Input: part model. Units: mm. Frame: model coordinates. Face numbers are marked on the shaded views. A direction names the side the tool comes from. Round coordinates to 2 decimals unless told otherwise and drop trailing zeros. Loops run counter-clockwise (first coordinate to the right, second up) from the corner with the lowest first, then second, coordinate; pieces in that order, holes last. Notation, with made-up numbers: M -35.5,12.25 L 15.5,12.25 A18 ccw 15.5,24.25 Z; hole C 66,-17.5 d7. An arc over 180 degrees is marked long. Put each result on its own line as item: value. Start each with the question number.
1) Draft query along X for the marked faces 4, 5 and 6. Return one class per face: +X half, -X half, draft (parallel to the pull), parting line (faces both ways), or undercut.
2) Reachability of the marked faces 1, 2 and 3 from +Z, -Z, +X, -X, +Y, -Y: full face, straight path, thin tool, end or side. Return the list, or none.
3) Section B-B on y = -3. Output: boundary loops of the cut face in (x, z).
4) Line query: probe 1 along Z at (x, y) = (25, 2); probe 2 along X at (y, z) = (1.5, -1.25); probe 3 along Y at (x, z) = (0, -3). Output: solid intervals per line, ascending.
5) Pin query (flat end, axial travel): pin 1 (3 mm diameter, centred on x = 12, z = 1.5, fed in from -Y); pin 2 (9.5 mm diameter, centred on x = 52, y = -11, fed in from -Z); pin 3 (2 mm diameter, centred on y = -16, z = 1, fed in from -X); pin 4 (1 mm diameter, centred on x = 76, y = -10, fed in from -Z). Return the tip coordinate at first contact, or that it passes through.
6) Section C-C on x = -25. Output: boundary loops of the cut face in (y, z), plus the area to 3 significant figures.
7) Section A-A on z = 2.5. Output: boundary loops of the cut face in (x, y), plus the area to 3 significant figures.
8) Section D-D on x = 88.5. Output: boundary loops of the cut face in (y, z), plus the area to 3 significant figures.
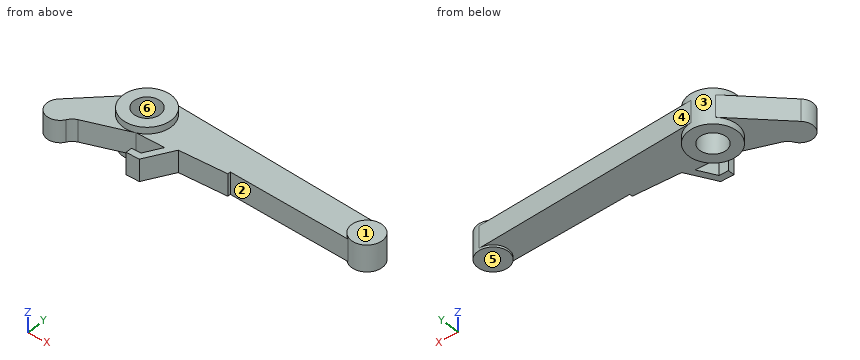
from build123d import *

# Parameters (mm, degrees)
SKETCH1_R               = 11
SKETCH1_R_2             = 6
BOSS_EXTRUDE1_DEPTH     = 8
SKETCH2_R               = 7
BOSS_EXTRUDE2_DEPTH     = 6
BOSS_EXTRUDE3_DEPTH     = 5
CUT_EXTRUDE1_DEPTH      = 112.742355901
CUT_EXTRUDE1_DEPTH_BACK = 112.742355901
SKETCH3_R               = 6


with BuildPart() as part:
    # Sketch1 → Boss-Extrude1 (new, symmetric)
    with BuildSketch(Plane.XY):
        Circle(SKETCH1_R)
        Circle(SKETCH1_R_2, mode=Mode.SUBTRACT)
    extrude(amount=BOSS_EXTRUDE1_DEPTH, both=True)



with BuildPart() as body_2:
    # Sketch2 → Boss-Extrude2 (new, symmetric)
    with BuildSketch(Plane.XY):
        with Locations((102, -3)):
            Circle(SKETCH2_R)
    extrude(amount=BOSS_EXTRUDE2_DEPTH, both=True)


with BuildPart() as part_1:
    add(part.part)

    add(body_2.part)  # Boss-Extrude3 merges body 2
    # Sketch2_3 → Boss-Extrude3 (add, symmetric)
    with BuildSketch(Plane.XY):
        with BuildLine():
            ThreePointArc((0.754140733, 10.974118268), (-3.77780396, 10.330933997), (-7.655588843, 7.898858112))
            Line((-7.655588843, 7.898858112), (-29.175775732, -12.958549415))
            ThreePointArc((-29.175775732, -12.958549415), (-28.687665444, -22), (-19.801298619, -20.262598212))
            ThreePointArc((-19.801298619, -20.262598212), (-18.446505094, -18.651187263), (-16.618471977, -17.606962351))
            Line((-16.618471977, -17.606962351), (3.695770356, -10.360563762))
            Line((3.695770356, -10.360563762), (16.576592604, -10.360563762))
            Line((16.576592604, -10.360563762), (12.165962036, -18))
            Line((12.165962036, -18), (7.898012843, -18))
            Line((7.898012843, -18), (7.898012843, -21))
            Line((7.898012843, -21), (13.898012843, -21))
            Line((13.898012843, -21), (21.138158023, -8.459700694))
            Line((21.138158023, -8.459700694), (42.898012843, -7.651891962))
            Line((42.898012843, -7.651891962), (42.898012843, -6.302949113))
            Line((42.898012843, -6.302949113), (98.5, -9.062177826))
            ThreePointArc((98.5, -9.062177826), (95.304638828, -0.957418601), (102.479907739, 3.983529807))
            Line((102.479907739, 3.983529807), (0.754140733, 10.974118268))
        make_face()
    extrude(amount=BOSS_EXTRUDE3_DEPTH, both=True)

    # Sketch3 → Cut-Extrude1 (cut, two sides: drawn at the far end of the back side and taken through both)
    with BuildSketch(Plane.XY.offset(-CUT_EXTRUDE1_DEPTH_BACK)):
        Circle(SKETCH3_R)
    extrude(amount=CUT_EXTRUDE1_DEPTH + CUT_EXTRUDE1_DEPTH_BACK, mode=Mode.SUBTRACT)


solid = part_1.part
Geometry results:
1. face 4: +X half
1. face 5: draft
1. face 6: undercut
2. face 1: +Z, +X, +Y, -Y
2. face 2: +Z, -Z, -Y
2. face 3: none
3. outline: M -18.9,-5 L -10.58,-5 L -10.58,-8 L -5.2,-8 L -5.2,8 L -10.58,8 L -10.58,5 L -18.9,5 Z; M 5.2,-8 L 10.58,-8 L 10.58,-5 L 95,-5 L 95,-6 L 109,-6 L 109,6 L 95,6 L 95,5 L 10.58,5 L 10.58,8 L 5.2,8 Z
4. probe 1: z = -5 to 5
4. probe 2: x = -14.26 to -5.81, 5.81 to 107.36
4. probe 3: y = -11.68 to -6, 6 to 11
5. pin 1: stops at y = -21
5. pin 2: stops at z = -5
5. pin 3: stops at x = -30.99
5. pin 4: passes through
6. outline: M -23.27,-5 L -8.91,-5 L -8.91,5 L -23.27,5 Z
6. area: 144 mm²
7. outline: M -29.18,-12.96 A6 ccw long -19.8,-20.26 A6 cw -16.62,-17.61 L 3.7,-10.36 L 16.58,-10.36 L 12.17,-18 L 7.9,-18 L 7.9,-21 L 13.9,-21 L 21.14,-8.46 L 42.9,-7.65 L 42.9,-6.3 L 98.5,-9.06 A7 ccw long 102.48,3.98 L 0.75,10.97 A11 ccw -7.66,7.9 Z; hole C 0,0 d12
7. area: 2,180 mm²
8. outline: M -8.57,-5 L 4.94,-5 L 4.94,5 L -8.57,5 Z
8. area: 135 mm²
